Geometry check sheet. Reference: the model listing, model coordinates, mm. Coordinates: 2 decimals unless noted, no trailing zeros. Loops run counter-clockwise (first coordinate to the right, second up) from the corner with the lowest first, then second, coordinate; pieces in that order, holes last.
Autodesk Inventor part; units mm, degrees
ref_plane "YZ Plane" through (0, 0, 0) normal (1, 0, 0) x (0, 1, 0)
ref_plane "XZ Plane" through (0, 0, 0) normal (0, 1, 0) x (-1, 0, 0)
ref_plane "XY Plane" through (0, 0, 0) normal (0, 0, 1) x (1, 0, 0)
sketch "スケッチ1" plane through (0, 0, 0) normal (0, 0, 1) x (1, 0, 0)
  line L0 (-90, -67.5) -> (90, -67.5)
  line L1 (90, -67.5) -> (90, 70)
  line L2 (90, 70) -> (-90, 70)
  line L3 (-90, 70) -> (-90, -67.5)
  point P0 (0, 0)
  point P1 (-29.0861, -67.5)
  dimension "d37" = 90
  dimension "d38" = 70
  dimension "d40" = 90
  dimension "d41" = 67.5
extrude "プレート1" add sketch "スケッチ1" along normal blind 2
sketch "スケッチ2" plane through (0, 0, 2) normal (0, 0, 1) x (1, 0, 0)
  circle A0 centre (0, 0) radius 45.5
  dimension "d5" = 91
extrude "押し出し1" cut sketch "スケッチ2" against normal blind 10
sketch "スケッチ3" plane through (0, 0, 2) normal (0, 0, 1) x (1, 0, 0)
  circle A0 centre (0, 0) radius 62.5
  point P0 (-16.1762, 60.3704)
  point P1 (-44.1942, 44.1942)
  point P2 (-60.3704, 16.1762)
  point P3 (-60.3704, -16.1762)
  point P4 (-44.1942, -44.1942)
  point P5 (-16.1762, -60.3704)
  point P6 (16.1762, -60.3704)
  point P7 (44.1942, -44.1942)
  point P8 (60.3704, -16.1762)
  point P9 (60.3704, 16.1762)
  point P10 (44.1942, 44.1942)
  point P11 (16.1762, 60.3704)
  dimension "d8" = 125
  dimension "d11" = 360
  dimension "d20" = 0
hole "穴1" at (-16.1762, 60.3704, 2) at (-44.1942, 44.1942, 2) at (-60.3704, 16.1762, 2) at (-60.3704, -16.1762, 2) at (-44.1942, -44.1942, 2) at (-16.1762, -60.3704, 2) at (16.1762, -60.3704, 2) at (44.1942, -44.1942, 2) at (60.3704, -16.1762, 2) at (60.3704, 16.1762, 2) at (44.1942, 44.1942, 2) at (16.1762, 60.3704, 2) direction (0, 0, -1) diameter 4.3 end through all
fillet "コーナーR2" radius 10 2 edges at (-90, 70, 1) (90, 70, 1)
sketch "スケッチ5" plane through (0, 0, 2) normal (0, 0, 1) x (1, 0, 0)
  arc A0 (-80, 70) -> (-90, 60) centre (-80, 60) ccw
  arc A1 (90, 60) -> (80, 70) centre (80, 60) ccw
  point P0 (0, 0)
hole "穴2" at (-80, 60, 2) at (80, 60, 2) direction (0, 0, -1) diameter 3.2 end through all
sketch "スケッチ7" plane through (0, 0, 2) normal (0, 0, 1) x (1, 0, 0)
  circle A0 centre (0, 0) radius 45.5
  circle A1 centre (0, 0) radius 67.5
  line L0 (90, -67.5) -> (-90, -67.5)
  line L1 (-90, -67.5) -> (-90, 60)
  line L2 (-90, -67.5) -> (-67.5, -67.5)
  line L3 (-67.5, -67.5) -> (-67.5, 50)
  line L4 (-67.5, 50) -> (-90, 50)
  line L5 (-90, 50) -> (-90, -67.5)
  line L6 (90, -67.5) -> (67.5, -67.5)
  line L7 (67.5, -67.5) -> (67.5, 50)
  line L8 (67.5, 50) -> (90, 50)
  line L9 (90, 50) -> (90, -67.5)
  line L10 (-80, 70) -> (80, 70)
  point P0 (67.5, 0)
  point P1 (0, -67.5)
  point P2 (-67.5, 0)
  dimension "d56" = 20
  dimension "d57" = 20
extrude "押し出し4" cut sketch "スケッチ7" against normal blind 10 contours L7 L0 A1 | L7 L8 L9 L0 | A1 L0 L3 | L3 L0 L1 L4
fillet "コーナーR4" radius 5 2 edges at (-67.5, 50, 1) (67.5, 50, 1)
sketch "スケッチ9" plane through (0, 0, 2) normal (0, 0, 1) x (1, 0, 0)
  circle A0 centre (0, 0) radius 45.5
  circle A1 centre (0, 0) radius 41.5
  line L0 (0, 0) -> (-11.7763, 43.9496)
  line L1 (11.7763, 43.9496) -> (0, 0)
  line L2 (0, 97.5) -> (0, -95)
  point P0 (-10.741, 40.0859)
  point P1 (10.741, 40.0859)
  dimension "d76" = 4
  dimension "d77" = 15
  dimension "d78" = 15
extrude "押し出し5" add sketch "スケッチ9" against normal up to surface (2 mm away) contours L1 A1 L2 A0 | L2 A1 L0 A0 picked at (5.1612, 43.8259) picked at (-6.3577, 43.6684)
fillet "コーナーR5" radius 1 4 edges at (10.741, 40.0859, 1) (-10.741, 40.0859, 1) (-11.7763, 43.9496, 1) (11.7763, 43.9496, 1)
equation "\"d18\" = Thickness"
equation "\"d47\" = Thickness"
equation "\"d2\" = Thickness"
equation "\"BendRadius\" = Thickness"
equation "\"BendReliefWidth\" = Thickness"
equation "\"BendReliefDepth\" = 0.5 * Thickness"
equation "\"CornerReliefSize\" = 4 * Thickness"
equation "\"MinimumRemnant\" = 2 * Thickness"
equation "\"TransitionRadius\" = BendRadius"
equation "\"JacobiRadiusSize\" = BendRadius"
equation "\"GapSize\" = Thickness"
properties part number "base4" material "CFRP"
(1) Sectioned sample at B-B on y = 4. Record the cut outline in (x, z).
Findings:
outline: (-67.5, 0) - (-45.32, 0) - (-45.32, 2) - (-67.5, 2) - close; (45.32, 0) - (67.5, 0) - (67.5, 2) - (45.32, 2) - close
(2) Scan lines: L1, parallel to X at y = 60, z = 1.35; L2, parallel to Y at x = -15, z = 1.65; L3, parallel to X at y = 1, z = 1.55. Record each from-to range of solid material in increasing order.
Findings:
L1: x = -90 to -81.6, -78.4 to -18.29, -14.06 to 14.06, 18.29 to 78.4, 81.6 to 90
L2: y = -65.81 to -62.17, -58.57 to -42.96, 42.96 to 58.57, 62.17 to 70
L3: x = -67.5 to -45.49, 45.49 to 67.5
(3) Sectioned sample at D-D on y = -52.5. Record the cut outline in (x, z).
Findings:
outline: (-42.43, 0) - (42.43, 0) - (42.43, 2) - (-42.43, 2) - close
(4) Sectioned sample at A-A on x = 0. Record the cut outline in (y, z).
Findings:
outline: (-67.5, 0) - (-45.5, 0) - (-45.5, 2) - (-67.5, 2) - close; (41.5, 0) - (70, 0) - (70, 2) - (41.5, 2) - close
(5) Gauge pin test, flat ends, axial feed: pin 1 Ø5 at (x, y) = (44.19, -44.19) entering from +Z; pin 2 Ø1 at (y, z) = (19, 1) entering from -X. Record the tip position at first contact, or that the pin passes through.
Findings:
pin 1: stops at z = 2
pin 2: stops at x = -67.5
(6) Sectioned sample at C-C on z = 1.2. State how many separate pieces and enclosed holes the cut face has, and give its area (3 significant figures).
Findings:
separate pieces: 1
enclosed holes: 15
area: 10,900 mm2
